from build123d import *

# Parameters (mm, degrees)
BOSS_EXTRUDE1_DEPTH                             = 50
CSK_FOR_M3_FLAT_HEAD_MACHINE_SCREW1_D           = 3.4
CSK_FOR_M3_FLAT_HEAD_MACHINE_SCREW1_CSINK_D     = 6.3
CSK_FOR_M3_FLAT_HEAD_MACHINE_SCREW1_CSINK_ANGLE = 90
SKETCH8_R                                       = 11.15
CUT_EXTRUDE1_DEPTH                              = 41
F_3_0_3_DIAMETER_HOLE1_D                        = 3
CHAMFER1_SIZE                                   = 3
SKETCH14_W                                      = 6
SKETCH14_H                                      = 6
BOSS_EXTRUDE2_DEPTH                             = 3
F_3_0_3_DIAMETER_HOLE2_D                        = 3


with BuildPart() as part:
    # Sketch2 → Boss-Extrude1 (new body)
    with BuildSketch(Plane.XY):
        Polygon((0, 0), (0, 37), (-50, 37), (-50, 0), (-70, 0), (-70, 5), (-55, 5), (-55, 42), (-50, 42), (5, 42), (5, 5), (20, 5), (20, 0), align=None)
    extrude(amount=BOSS_EXTRUDE1_DEPTH)

    # CSK for M3 Flat Head Machine Screw1 (through all)
    with Locations(Plane(origin=(0, 5, 0), x_dir=(1, 0, 0), z_dir=(0, 1, 0))):
        with Locations((-62.5, -10), (-62.5, -40), (12.5, -40), (12.5, -10)):
            CounterSinkHole(CSK_FOR_M3_FLAT_HEAD_MACHINE_SCREW1_D / 2, CSK_FOR_M3_FLAT_HEAD_MACHINE_SCREW1_CSINK_D / 2, counter_sink_angle=CSK_FOR_M3_FLAT_HEAD_MACHINE_SCREW1_CSINK_ANGLE)

    # Sketch8 → Cut-Extrude1 (cut)
    with BuildSketch(Plane(origin=(0, 42, 0), x_dir=(1, 0, 0), z_dir=(0, 1, 0))):
        with Locations(Location((-25, -25, 0), (0, 0, 180))):
            Circle(SKETCH8_R)
    extrude(amount=-CUT_EXTRUDE1_DEPTH, mode=Mode.SUBTRACT)

    # Ø3.0 (3) Diameter Hole1 (through all)
    with Locations(Plane(origin=(0, 42, 0), x_dir=(1, 0, 0), z_dir=(0, 1, 0))):
        with Locations((-40.5, -40.5), (-40.5, -9.5), (-9.5, -9.5), (-9.5, -40.5)):
            Hole(F_3_0_3_DIAMETER_HOLE1_D / 2)

    # Chamfer1
    chamfer1_edges = [part.edges().sort_by_distance(p)[0] for p in [
        (-70, 5, 25),
        (20, 5, 25),
    ]]
    chamfer(chamfer1_edges, length=CHAMFER1_SIZE)

    # Sketch14 → Boss-Extrude2 (add)
    with BuildSketch(Plane(origin=(0, 42, 0), x_dir=(1, 0, 0), z_dir=(0, 1, 0))):
        with Locations((-52, 3)):
            Rectangle(SKETCH14_W, SKETCH14_H)
        with Locations((-52, -53)):
            Rectangle(SKETCH14_W, SKETCH14_H)
        with Locations((2, 3)):
            Rectangle(SKETCH14_W, SKETCH14_H)
        with Locations((2, -53)):
            Rectangle(SKETCH14_W, SKETCH14_H)
    extrude(amount=-BOSS_EXTRUDE2_DEPTH)

    # Ø3.0 (3) Diameter Hole2 (through all)
    with Locations(Plane(origin=(0, 42, 0), x_dir=(1, 0, 0), z_dir=(0, 1, 0))):
        with Locations((-52, 3), (2, 3), (2, -53), (-52, -53)):
            Hole(F_3_0_3_DIAMETER_HOLE2_D / 2)


solid = part.part
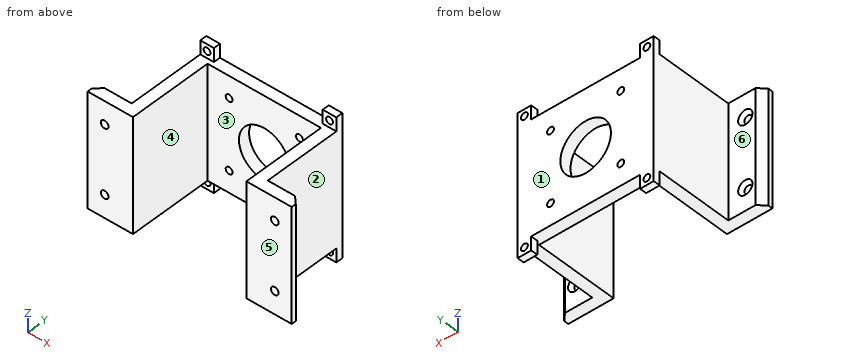
Input: part model. Units: mm. Frame: model coordinates. Face numbers are marked on the shaded views. A direction names the side the tool comes from. Round coordinates to 2 decimals unless told otherwise and drop trailing zeros. Loops run counter-clockwise (first coordinate to the right, second up) from the corner with the lowest first, then second, coordinate; pieces in that order, holes last. Notation, with made-up numbers: (75, -8.75) -> (129, -8.75) arc R3 ccw to (129, -4.75) -> close; hole circle Ø4 at (24.25, 0.25). An arc over 180 degrees is marked (long way). Answer as a JSON object with one key per item and string values. Group by question number.
1) Pin query (flat end, axial travel): pin 1 (11 mm diameter, centred on y = 30, z = 33.5, fed in from +X); pin 2 (4 mm diameter, centred on x = -62.5, z = 40, fed in from +Y); pin 3 (2 mm diameter, centred on x = 12.5, z = 10, fed in from -Y); pin 4 (9.5 mm diameter, centred on x = -61.5, z = 23, fed in from +Y). Return the tip coordinate at first contact, or that it passes through.
2) Section query B-B on y = 13. Output: boundary loops of the cut face in (x, z), plus the area to 3 significant figures.
3) Section query A-A on x = -9.5. Output: boundary loops of the cut face in (y, z).
4) Draft query along X for the marked faces 1, 2 and 3. Return one class per face: +X half, -X half, draft (parallel to the pull), parting line (faces both ways), or undercut.
5) Ray query, L1, parallel to X at y = 41, z = 53; L2, parallel to X at y = 1, z = 40; L3, parallel to Z at x = -62.5, y = 0.9. Return the intervals inside material, ascending.
6) Section query D-D on x = -21. Output: boundary loops of the cut face in (y, z), plus the area to 3 significant figures.
7) Section query C-C on z = 49. Output: boundary loops of the cut face in (x, y), plus the area to 3 significant figures.
8) Reachability of the marked faces 4, 5 and 6 from +Z, -Z, +X, -X, +Y, -Y: full face, straight path, thin tool, end or side. Return the list, or none.
Reply:
{
 "1": {"pin 1": "stops at x = 5", "pin 2": "stops at y = 3.85", "pin 3": "passes through", "pin 4": "stops at y = 5"},
 "2": {"outline": "(-55, 0) -> (-50, 0) -> (-50, 50) -> (-55, 50) -> close; (0, 0) -> (5, 0) -> (5, 50) -> (0, 50) -> close", "area": "500 mm2"},
 "3": {"outline": "(37, 0) -> (42, 0) -> (42, 8) -> (37, 8) -> close; (37, 11) -> (42, 11) -> (42, 39) -> (37, 39) -> close; (37, 42) -> (42, 42) -> (42, 50) -> (37, 50) -> close"},
 "4": {"face 1": "draft", "face 2": "+X half", "face 3": "undercut"},
 "5": {"L1": "x = -55 to -53.5, -50.5 to -49, -1 to 0.5, 3.5 to 5", "L2": "x = -70 to -64.2, -60.8 to -50, 0 to 10.8, 14.2 to 20", "L3": "z = 0 to 8.3, 11.7 to 38.3, 41.7 to 50"},
 "6": {"outline": "(37, 0) -> (42, 0) -> (42, 14.59) -> (37, 14.59) -> close; (37, 35.41) -> (42, 35.41) -> (42, 50) -> (37, 50) -> close", "area": "146 mm2"},
 "7": {"outline": "(-70, 0) -> (-50, 0) -> (-50, 37) -> (0, 37) -> (0, 0) -> (20, 0) -> (20, 2) -> (17, 5) -> (5, 5) -> (5, 42) -> (-55, 42) -> (-55, 5) -> (-67, 5) -> (-70, 2) -> close", "area": "811 mm2"},
 "8": {"face 4": "+Z, -Z, -Y", "face 5": "+Z, -Z, +X, -X, -Y", "face 6": "+Z, -Z, -X, +Y"}
}
